Input: part model. Units: mm. Frame: model coordinates. A direction names the side the tool comes from. Give positions to 0.01 mm unless a question says otherwise; leave off trailing zeros. Order: outer loops, then holes, each group sorted by start corner. A loop starts at its lowest first (then second) coordinate and runs counter-clockwise, first axis right, second up. Notation, with made-up numbers: (47, 54) - (98, 54) arc R22 cw to (98, 74) - close; hole circle Ø3 at (18, -19.75). An arc over 180 degrees is marked (long way). Answer in a Markdown table with one row per item. Add a question column.
from build123d import *

# Parameters (mm, degrees)
SKETCH1_R           = 2.75
BOSS_EXTRUDE1_DEPTH = 5
BOSS_EXTRUDE2_DEPTH = 35
SKETCH2_3_W         = 20
SKETCH2_3_H         = 20
BOSS_EXTRUDE3_DEPTH = 200


with BuildPart() as part:
    # Sketch1 → Boss-Extrude1 (new body)
    with BuildSketch(Plane(origin=(0, 0, 0), x_dir=(1, 0, 0), z_dir=(0, 1, 0))):
        with BuildLine():
            Line((-150, 0), (-150, 100))
            Line((-150, 100), (150, 100))
            Line((150, 100), (150, 0))
            ThreePointArc((150, 0), (0, -150), (-150, 0))
        make_face()
        with Locations((135, 0)):
            Circle(SKETCH1_R, mode=Mode.SUBTRACT)
        with Locations((134.486284242, -11.766025271)):
            Circle(SKETCH1_R, mode=Mode.SUBTRACT)
        with Locations((132.949046657, -23.442503985)):
            Circle(SKETCH1_R, mode=Mode.SUBTRACT)
        with Locations((130.399986549, -34.940571089)):
            Circle(SKETCH1_R, mode=Mode.SUBTRACT)
        with Locations((126.858503806, -46.172719349)):
            Circle(SKETCH1_R, mode=Mode.SUBTRACT)
        with Locations((122.35155125, -57.053465335)):
            Circle(SKETCH1_R, mode=Mode.SUBTRACT)
        with Locations((116.913429511, -67.5)):
            Circle(SKETCH1_R, mode=Mode.SUBTRACT)
        with Locations((110.585525979, -77.432818907)):
            Circle(SKETCH1_R, mode=Mode.SUBTRACT)
        with Locations((103.415999821, -86.776327308)):
            Circle(SKETCH1_R, mode=Mode.SUBTRACT)
        with Locations((95.45941546, -95.45941546)):
            Circle(SKETCH1_R, mode=Mode.SUBTRACT)
        with Locations((86.776327308, -103.415999821)):
            Circle(SKETCH1_R, mode=Mode.SUBTRACT)
        with Locations((77.432818907, -110.585525979)):
            Circle(SKETCH1_R, mode=Mode.SUBTRACT)
        with Locations((67.5, -116.913429511)):
            Circle(SKETCH1_R, mode=Mode.SUBTRACT)
        with Locations((57.053465335, -122.35155125)):
            Circle(SKETCH1_R, mode=Mode.SUBTRACT)
        with Locations((46.172719349, -126.858503806)):
            Circle(SKETCH1_R, mode=Mode.SUBTRACT)
        with Locations((34.940571089, -130.399986549)):
            Circle(SKETCH1_R, mode=Mode.SUBTRACT)
        with Locations((23.442503985, -132.949046657)):
            Circle(SKETCH1_R, mode=Mode.SUBTRACT)
        with Locations((11.766025271, -134.486284242)):
            Circle(SKETCH1_R, mode=Mode.SUBTRACT)
        with Locations((0, -135)):
            Circle(SKETCH1_R, mode=Mode.SUBTRACT)
        with Locations((-11.766025271, -134.486284242)):
            Circle(SKETCH1_R, mode=Mode.SUBTRACT)
        with Locations((-23.442503985, -132.949046657)):
            Circle(SKETCH1_R, mode=Mode.SUBTRACT)
        with Locations((-34.940571089, -130.399986549)):
            Circle(SKETCH1_R, mode=Mode.SUBTRACT)
        with Locations((-46.172719349, -126.858503806)):
            Circle(SKETCH1_R, mode=Mode.SUBTRACT)
        with Locations((-57.053465335, -122.35155125)):
            Circle(SKETCH1_R, mode=Mode.SUBTRACT)
        with Locations((-67.5, -116.913429511)):
            Circle(SKETCH1_R, mode=Mode.SUBTRACT)
        with Locations((-77.432818907, -110.585525979)):
            Circle(SKETCH1_R, mode=Mode.SUBTRACT)
        with Locations((-86.776327308, -103.415999821)):
            Circle(SKETCH1_R, mode=Mode.SUBTRACT)
        with Locations((-95.45941546, -95.45941546)):
            Circle(SKETCH1_R, mode=Mode.SUBTRACT)
        with Locations((-103.415999821, -86.776327308)):
            Circle(SKETCH1_R, mode=Mode.SUBTRACT)
        with Locations((-110.585525979, -77.432818907)):
            Circle(SKETCH1_R, mode=Mode.SUBTRACT)
        with Locations((-116.913429511, -67.5)):
            Circle(SKETCH1_R, mode=Mode.SUBTRACT)
        with Locations((-122.35155125, -57.053465335)):
            Circle(SKETCH1_R, mode=Mode.SUBTRACT)
        with Locations((-126.858503806, -46.172719349)):
            Circle(SKETCH1_R, mode=Mode.SUBTRACT)
        with Locations((-130.399986549, -34.940571089)):
            Circle(SKETCH1_R, mode=Mode.SUBTRACT)
        with Locations((-132.949046657, -23.442503985)):
            Circle(SKETCH1_R, mode=Mode.SUBTRACT)
        with Locations((-134.486284242, -11.766025271)):
            Circle(SKETCH1_R, mode=Mode.SUBTRACT)
        with Locations((-135, 0)):
            Circle(SKETCH1_R, mode=Mode.SUBTRACT)
    extrude(amount=BOSS_EXTRUDE1_DEPTH)

    # Sketch2 → Boss-Extrude2 (add)
    with BuildSketch(Plane(origin=(0, 5, 0), x_dir=(1, 0, 0), z_dir=(0, 1, 0))):
        Polygon((150, 25), (150, 50), (120, 50), (120, 25), (125, 25), (125, 45), (145, 45), (145, 25), align=None)
    extrude(amount=BOSS_EXTRUDE2_DEPTH)

    # Sketch2<3> → Boss-Extrude3 (add)
    with BuildSketch(Plane(origin=(0, 5, 0), x_dir=(1, 0, 0), z_dir=(0, 1, 0))):
        with Locations((135, 35)):
            Rectangle(SKETCH2_3_W, SKETCH2_3_H)
    extrude(amount=BOSS_EXTRUDE3_DEPTH)


solid = part.part
Q1. Section A-A, the plane y = 190.5. Return loops of the section in (x, z), then the cut area to 3 significant figures.
Q2. Section B-B, the plane z = -62.5. Return loops of the section in (x, y).
Q3. Contact query for flat-ended pins moving along their axis: P1, Ø3, axis at y = 60.5, z = -26.5, coming from the +X side; P2, Ø6, axis at x = -106.5, z = 89.5, coming from the +Y side; P3, Ø3.5, axis at x = -57.05, z = 122.35, coming from the -Y side; P4, Ø10, axis at x = 133.5, y = 139.5, coming from the -Z side. Output: stop coordinate, or through.
Q4. Access query for faces 1 (the flat face through (125, 121, -35)), 2 (the flat face through (135, 22, -50)), 3 (the flat face through (145, 121, -35)), 4 (the flat face through (135, 205, -35)), 5 (the flat face through (135, 104, -25)). Directions: +Z, -Z, +X, -X, +Y, -Y. A direction counts if a zero-diameter tool reaches every point of the face in a straight line with its end or side. Return the directions, or none.
Q5. Line query: probe 1 along Y at (x, z) = (48, 35.5); probe 2 along Z at (x, y) = (125.5, 88); probe 3 along X at (y, z) = (119, -37). Output: solid intervals per line, ascending.
Computed:
| question | item | result |
|---|---|---|
| 1 | outline | (125, -45) - (145, -45) - (145, -25) - (125, -25) - close |
| 1 | area | 400 mm^2 |
| 2 | outline | (-150, 0) - (150, 0) - (150, 5) - (-150, 5) - close |
| 3 | P1 | stops at x = 145 |
| 3 | P2 | stops at y = 5 |
| 3 | P3 | passes through |
| 3 | P4 | stops at z = -45 |
| 4 | face 1 | +Z, -Z, -X, +Y |
| 4 | face 2 | -Z, +X, -X, +Y |
| 4 | face 3 | +Z, -Z, +X, +Y |
| 4 | face 4 | +Z, -Z, +X, -X, +Y |
| 4 | face 5 | +Z, +X, -X, +Y |
| 5 | probe 1 | y = 0 to 5 |
| 5 | probe 2 | z = -45 to -25 |
| 5 | probe 3 | x = 125 to 145 |
